Autodesk Inventor part; units mm, degrees
ref_plane "YZ Plane" through (0, 0, 0) normal (1, 0, 0) x (0, 1, 0)
ref_plane "XZ Plane" through (0, 0, 0) normal (0, 1, 0) x (-1, 0, 0)
ref_plane "XY Plane" through (0, 0, 0) normal (0, 0, 1) x (1, 0, 0)
sketch "Sketch1" plane through (0, 0, 0) normal (1, 0, 0) x (0, 1, 0)
  circle A0 centre (0, 0) radius 6
  circle A1 centre (0, 0) radius 3
  dimension "d0" = 12
  dimension "d1" = 6
extrude "Extrusion1" add sketch "Sketch1" along normal blind 4
sketch "Sketch2" plane through (0, 0, 0) normal (-1, 0, 0) x (0, 0, 1)
  circle A0 centre (0, 0) radius 6
  circle A1 centre (0, 0) radius 3
  circle A2 centre (0, 0) radius 5.2
  circle A3 centre (0, 0) radius 3.8
  dimension "d4" = 0.8
  dimension "d5" = 0.8
extrude "Extrusion2" cut sketch "Sketch2" against normal blind 0.1 contours A2
sketch "Sketch3" plane through (4, 0, 0) normal (1, 0, 0) x (0, 0, -1)
  circle A0 centre (0, 0) radius 6
  circle A1 centre (0, 0) radius 5.2
  circle A2 centre (0, 0) radius 3.8
extrude "Extrusion3" cut sketch "Sketch3" against normal blind 0.1 contours A1
properties part number "MR126ZZ-6x12x4mm" material "Stainless Steel"
Geometry: final body of the model. Coordinates: model frame, mm. A direction names the side the tool comes from. Round coordinates to 2 decimals unless told otherwise and drop trailing zeros. Loops run counter-clockwise (first coordinate to the right, second up) from the corner with the lowest first, then second, coordinate; pieces in that order, holes last. Notation, with made-up numbers: M 27.25,67 L 72.25,67 A27 cw 72.25,101 Z; hole C -1.75,-20.5 d1. An arc over 180 degrees is marked long. One line per question, with ' | ' between items.
(1) Cut plane A-A on z = 0. Return the cut outline in (x, y).
Check result:
outline: M 0,-6 L 4,-6 L 4,-5.2 L 3.9,-5.2 L 3.9,-3.8 L 4,-3.8 L 4,-3 L 0,-3 L 0,-3.8 L 0.1,-3.8 L 0.1,-5.2 L 0,-5.2 Z; M 0,3 L 4,3 L 4,3.8 L 3.9,3.8 L 3.9,5.2 L 4,5.2 L 4,6 L 0,6 L 0,5.2 L 0.1,5.2 L 0.1,3.8 L 0,3.8 Z
(2) Material intervals for line 1 along Z through (x, y) = (2, 0); line 2 along Z through (x, y) = (3.7, -2.25); line 3 along X through (y, z) = (-1.5, -3.75), sorted ascending. Write a range as from..to.
Check result:
line 1: z = -6..-3, 3..6 | line 2: z = -5.56..-1.98, 1.98..5.56 | line 3: x = 0.1..3.9
(3) Cut plane D-D on x = 3.4. Return the cut outline in (y, z), plus the area to 3 significant figures.
Check result:
outline: C 0,0 d12; hole C 0,0 d6 | area: 84.8 mm2
(4) Pull-direction query (Y, two-part tool) for faces 1 (the cylindrical face through (2, -3, 0)), 2 (the flat face through (3.9, -4, 0)), 3 (the cylindrical face through (2, -6, 0)), 4 (the flat face through (0, -2, 5)); classes: +Y half, -Y half, draft (parallel to the pull), parting line (faces both ways), or undercut.
Check result:
face 1: undercut | face 2: undercut | face 3: parting line | face 4: draft
(5) Contact query for a flat-ended pin moving along its axis: P1, Ø2, axis at x = 1.5, y = 3, coming from the +Z side. Output: stop coordinate, or through.
Check result:
P1: stops at z = 5.66
(6) Access query for faces 5 (the flat face through (4, -2, 5)), 6 (the flat face through (0.1, -4, 0)). Directions: +Z, -Z, +X, -X, +Y, -Y. A direction counts if a zero-diameter tool reaches every point of the face in a straight line with its end or side. Return the directions, or none.
Check result:
face 5: +Z, -Z, +X, +Y, -Y | face 6: -X
(7) Cut plane C-C on y = -3.5. Return the cut outline in (x, z).
Check result:
outline: M 0,-4.87 L 4,-4.87 L 4,-3.85 L 3.9,-3.85 L 3.9,-1.48 L 4,-1.48 L 4,1.48 L 3.9,1.48 L 3.9,3.85 L 4,3.85 L 4,4.87 L 0,4.87 L 0,3.85 L 0.1,3.85 L 0.1,1.48 L 0,1.48 L 0,-1.48 L 0.1,-1.48 L 0.1,-3.85 L 0,-3.85 Z
